```python
from build123d import *

# Parameters (mm, degrees)
F0_W      = 15.494
F0_H      = 15.494
F1_DEPTH  = 7.747
F3_DEPTH  = 10.16
F5_DEPTH  = 7.366
F6_W      = 15.494
F6_H      = 7.747
F7_DEPTH  = 16.002
F8_W      = 8.001
F8_H      = 7.747
F9_DEPTH  = 7.62
F11_DEPTH = 7.747


with BuildPart() as f1:
    # F0 (on Front) → F1 (new body, symmetric)
    with BuildSketch(Plane.XZ):
        Rectangle(F0_W, F0_H)
    extrude(amount=F1_DEPTH, both=True)

    # F2 (on face) → F3 (join)
    with BuildSketch(Plane.XZ.offset(7.747)):
        Polygon((-7.747, -0.381), (-7.747, -7.747), (-0.889, -7.747), align=None)
    extrude(amount=F3_DEPTH)

    # F4 (on face) → F5 (join)
    with BuildSketch(Plane.XZ.offset(17.907)):
        Polygon((0, -7.747), (0, 7.747), (-7.747, 7.747), (-7.747, -7.747), (-0.889, -7.747), align=None)
    extrude(amount=F5_DEPTH)

    # F6 (on face) → F7 (join)
    with BuildSketch(Plane.YZ.offset(7.747)):
        with Locations((0, -3.8735)):
            Rectangle(F6_W, F6_H)
    extrude(amount=F7_DEPTH)

    # F8 (on face) → F9 (join)
    with BuildSketch(Plane.XY):
        with Locations((19.7485, -3.8735)):
            Rectangle(F8_W, F8_H)
    extrude(amount=F9_DEPTH)

    # F10 (on face) → F11 (join)
    with BuildSketch(Plane.XZ.offset(7.747)):
        Polygon((15.748, 7.62), (7.747, 0), (15.748, 0), align=None)
    extrude(amount=-F11_DEPTH)


solid = f1.part
```
Verification items for the finished model (mm, model axes). A direction names the side the tool comes from. Give positions to 0.01 mm unless a question says otherwise; leave off trailing zeros. Loops run counter-clockwise (first coordinate to the right, second up) from the corner with the lowest first, then second, coordinate; pieces in that order, holes last.
1. Section check D-D, the plane z = -2.75. Enter the section's corners in (x, y), then the cut area to 3 significant figures.
2. Section check B-B, the plane z = 2.25. Enter the section's corners in (x, y), then the cut area to 3 significant figures.
3. Go/stop test with flat-tipped pins: pin 1 Ø8 at (x, z) = (7, 6) entering from -Y; pin 2 Ø8.5 at (x, y) = (13, 5) entering from +Z; pin 3 Ø4 at (y, z) = (-10.5, -4) entering from +X. Record where each tip stops, or that it passes through.
4. Section check C-C, the plane x = -5. Enter the section's corners in (y, z).
5. Set-up check for faces 1 (the flat face through (-4.27, -12.756, -4.116)), 2 (the flat face through (0, -22, 0)), 3 (the flat face through (16, 4, 0)), 4 (the flat face through (11.8, -3.93, 3.86)), 5 (the flat face through (20, -4, 7.62)): record each of +Z, -Z, +X, -X, +Y, -Y from which the full face is reachable in a straight line by a thin tool's end or side.
6. Section check A-A, the plane y = -6.5. Enter the section's corners in (x, z), then the cut area to 3 significant figures.
7. Mould release check, pull along Y, two halves, no side actions. Record for faces 6 (the flat face through (-4, -17.907, 2)), 7 (the flat face through (8, -7.747, -2)), 8 (the flat face through (4, 7.747, -2)), 9 (the flat face through (4, -2, -7.747)): released by +Y, released by -Y, zero draft, split by the parting line, or undercut.
8. Thickness scan on line 1 (Y direction, x = -1, z = -2.75); line 2 (Y direction, x = 21.5, z = 2.25); line 3 (X direction, y = 5, z = 4.5). Record the ranges inside material, lowest first.
Geometry says:
1. outline: (-7.75, -25.27) - (0, -25.27) - (0, -17.91) - (-5.54, -17.91) - (-5.54, -7.75) - (23.75, -7.75) - (23.75, 7.75) - (-7.75, 7.75) - close
1. area: 567 mm2
2. outline: (-7.75, -25.27) - (0, -25.27) - (0, -17.91) - (-7.75, -17.91) - close; (-7.75, -7.75) - (7.75, -7.75) - (7.75, 7.75) - (-7.75, 7.75) - close; (10.11, -7.75) - (23.75, -7.75) - (23.75, 0) - (10.11, 0) - close
2. area: 403 mm2
3. pin 1: stops at y = -7.75
3. pin 2: stops at z = 0
3. pin 3: stops at x = -2.52
4. outline: (-25.27, -7.75) - (7.75, -7.75) - (7.75, 7.75) - (-7.75, 7.75) - (-7.75, -3.33) - (-17.91, -3.33) - (-17.91, 7.75) - (-25.27, 7.75) - close
5. face 1: +Z, +X
5. face 2: +Z, -Z, +X, -Y
5. face 3: +Z, +X, +Y
5. face 4: +Z, +Y, -Y
5. face 5: +Z, +X, +Y, -Y
6. outline: (-7.75, -7.75) - (23.75, -7.75) - (23.75, 7.62) - (15.75, 7.62) - (7.75, 0) - (7.75, 7.75) - (-7.75, 7.75) - close
6. area: 455 mm2
7. face 6: undercut
7. face 7: undercut
7. face 8: released by +Y
7. face 9: zero draft
8. line 1: y = -25.27 to -17.91, -7.75 to 7.75
8. line 2: y = -7.75 to 0
8. line 3: x = -7.75 to 7.75
